Model file for the job. Use its own axes, mm. Face numbers are marked on the shaded views. A direction names the side the tool comes from. Coordinates: 2 decimals unless noted, no trailing zeros. Loops run counter-clockwise (first coordinate to the right, second up) from the corner with the lowest first, then second, coordinate; pieces in that order, holes last.
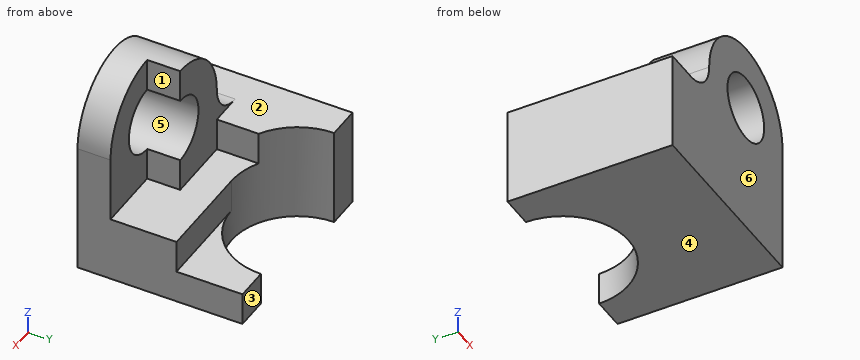
from build123d import *

# Parameters (mm, degrees)
BOSS_EXTRUDE1_DEPTH = 3
SKETCH2_W           = 2
SKETCH2_H           = 2
CUT_EXTRUDE14_DEPTH = 2
SKETCH6_W           = 1
SKETCH6_H           = 3.267949192
CUT_EXTRUDE16_DEPTH = 4
CUT_EXTRUDE17_DEPTH = 1
SKETCH9_R           = 1
BOSS_EXTRUDE2_DEPTH = 2
CUT_EXTRUDE18_DEPTH = 1


with BuildPart() as part:
    # Sketch1 → Boss-Extrude1 (new body)
    with BuildSketch(Plane.XY):
        with BuildLine():
            Line((-2, 0), (-3, 0))
            Line((-3, 0), (-3, -5))
            Line((-3, -5), (3, -5))
            Line((3, -5), (3, 0))
            Line((3, 0), (2, 0))
            ThreePointArc((2, 0), (0, -2), (-2, 0))
        make_face()
    extrude(amount=BOSS_EXTRUDE1_DEPTH)

    # Sketch2 → Cut-Extrude14 (cut)
    with BuildSketch(Plane(origin=(0, 0, 0), x_dir=(1, 0, 0), z_dir=(0, 1, 0))):
        with Locations((2, -2)):
            Rectangle(SKETCH2_W, SKETCH2_H)
    extrude(amount=-CUT_EXTRUDE14_DEPTH, mode=Mode.SUBTRACT)

    # Sketch6 → Cut-Extrude16 (cut)
    with BuildSketch(Plane(origin=(3, 0, 0), x_dir=(0, 0, -1), z_dir=(1, 0, 0))):
        with Locations((-2.5, -3.366025404)):
            Rectangle(SKETCH6_W, SKETCH6_H)
    extrude(amount=-CUT_EXTRUDE16_DEPTH, mode=Mode.SUBTRACT)

    # Sketch8 → Cut-Extrude17 (cut)
    with BuildSketch(Plane.XY.offset(2)):
        with BuildLine():
            Line((1, -2), (0, -2))
            ThreePointArc((0, -2), (0.51763809, -1.931851653), (1, -1.732050808))
            Line((1, -1.732050808), (1, -2))
        make_face()
    extrude(amount=-CUT_EXTRUDE17_DEPTH, mode=Mode.SUBTRACT)

    # Sketch9 → Boss-Extrude2 (add)
    with BuildSketch(Plane.XZ.offset(5)):
        with BuildLine():
            Line((3, 2), (3, 4))
            ThreePointArc((3, 4), (1, 6), (-1, 4))
            ThreePointArc((-1, 4), (-1.292893219, 3.292893219), (-2, 3))
            Line((-2, 3), (-1, 3))
            Line((-1, 3), (-1, 2))
            Line((-1, 2), (3, 2))
        make_face()
        with Locations((1, 4)):
            Circle(SKETCH9_R, mode=Mode.SUBTRACT)
    extrude(amount=-BOSS_EXTRUDE2_DEPTH)

    # Sketch10 → Cut-Extrude18 (cut)
    with BuildSketch(Plane(origin=(0, -3, 0), x_dir=(1, 0, 0), z_dir=(0, 1, 0))):
        with BuildLine():
            Line((1, -2), (1, -6))
            ThreePointArc((1, -6), (2.414213562, -5.414213562), (3, -4))
            Line((3, -4), (3, -2))
            Line((3, -2), (1, -2))
        make_face()
    extrude(amount=-CUT_EXTRUDE18_DEPTH, mode=Mode.SUBTRACT)


solid = part.part
Q1. Slice it at D-D (y = -3.6). List the corners of the cut face in (x, z).
Answers:
outline: (-3, 0) - (3, 0) - (3, 2) - (1, 2) - (1, 3) arc R1 cw to (1, 5) - (1, 6) arc R2 ccw to (-1, 4) arc R1 cw to (-2, 3) - (-3, 3) - close
Q2. Mould opens along Z. For the marked faces 4, 5 and 6 say: +Z half, -Z half, draft (parallel to the pull), parting line (faces both ways), or undercut.
Answers:
face 4: -Z half
face 5: undercut
face 6: draft
Q3. Slice it at C-C (y = -0.75). List the corners of the cut face in (x, z), and give its area (3 significant figures).
Answers:
outline: (-3, 0) - (-1.85, 0) - (-1.85, 3) - (-3, 3) - close; (1.85, 0) - (3, 0) - (3, 1) - (1.85, 1) - close
area: 4.58 mm2
Q4. Drill centre lines: line 1 (Z direction, x = 1, y = -4.3); line 2 (X direction, y = -4.4, z = 4); line 3 (X direction, y = -3.7, z = 4). Where is each one in solid material? Low to high.
Answers:
line 1: z = 0 to 3, 5 to 6
line 2: x = -1 to 0, 2 to 3
line 3: x = -1 to 0
Q5. Slice it at A-A (z = 3.65). List the corners of the cut face in (x, y), and give its area (3 significant figures).
Answers:
outline: (-1.06, -5) - (0.06, -5) - (0.06, -3) - (-1.06, -3) - close; (1.94, -5) - (3, -5) - (3, -4) - (1.94, -4) - close
area: 3.32 mm2
Q6. Which spindle directions (+Z, -Z, +X, -X, +Y, -Y) get a long thin tool onto all of the face, cutting with end or side? Do the marked faces 1, 2 and 3. Say none if no direction does.
Answers:
face 1: +Z, +X, +Y
face 2: +Z, -X, +Y
face 3: +Z, -Z, +X, -X, +Y
Q7. Flat gauge pins, fed straight in: P1, Ø1, axis at x = 1.5, y = -0.5, coming from the +Z side; P2, Ø0.5, axis at x = 1, z = 1.5, coming from the +Y side; P3, Ø0.6, axis at x = 2, z = 3, coming from the +Y side; P4, Ø1.5, axis at x = -2, z = 3.5, coming from the +Y side. Where does each tip first touch, or does it go through?
Answers:
P1: stops at z = 1
P2: stops at y = -2
P3: stops at y = -4
P4: stops at y = 0
Q8. Slice it at B-B (x = 1.15). List the corners of the cut face in (y, z), and give its area (3 significant figures).
Answers:
outline: (-5, 0) - (-1.64, 0) - (-1.64, 1) - (-2, 1) - (-2, 2) - (-4, 2) - (-4, 3.01) - (-5, 3.01) - close; (-5, 4.99) - (-4, 4.99) - (-4, 5.99) - (-5, 5.99) - close
area: 8.38 mm2
